```python
from build123d import *

# Parameters (mm, degrees)
SKETCH_1_W          = 100
SKETCH_1_H          = 90
EXTRUDE_1_DEPTH     = 125
SKETCH_4_W          = 100
SKETCH_4_H          = 83
CUT_EXTRUDE_3_DEPTH = 120
FILLET_4_R          = 5
CUT_EXTRUDE_4_DEPTH = 120
SKETCH_6_W          = 23
SKETCH_6_H          = 12.5
CUT_EXTRUDE_5_DEPTH = 2


with BuildPart() as part:
    # 스케치1 → 보스-돌출1 (new body)
    with BuildSketch(Plane(origin=(0, 0, 0), x_dir=(1, 0, 0), z_dir=(0, 1, 0))):
        Rectangle(SKETCH_1_W, SKETCH_1_H)
    extrude(amount=EXTRUDE_1_DEPTH)

    # 스케치4 → 컷-돌출3 (cut)
    with BuildSketch(Plane.XZ):
        with Locations((0, -3.5)):
            Rectangle(SKETCH_4_W, SKETCH_4_H)
    extrude(amount=-CUT_EXTRUDE_3_DEPTH, mode=Mode.SUBTRACT)

    # 필렛4
    fillet_4_edges = [part.edges().sort_by_distance(p)[0] for p in [
        (50, 62.5, 45),
        (-50, 62.5, 45),
        (-50, 122.5, -45),
        (50, 122.5, -45),
    ]]
    fillet(fillet_4_edges, radius=FILLET_4_R)

    # 스케치5 → 컷-돌출4 (cut)
    with BuildSketch(Plane(origin=(0, 0, 38), x_dir=(-1, 0, 0), z_dir=(0, 0, -1))):
        with BuildLine():
            Line((26.25, 63), (28.26707195, 63))
            ThreePointArc((28.26707195, 63), (40, 60), (28.26707195, 57))
            Line((28.26707195, 57), (26.25, 57))
            ThreePointArc((26.25, 57), (23.25, 60), (26.25, 63))
        make_face()
    extrude(amount=-CUT_EXTRUDE_4_DEPTH, mode=Mode.SUBTRACT)

    # 스케치6 → 컷-돌출5 (cut)
    with BuildSketch(Plane(origin=(0, 0, 38), x_dir=(-1, 0, 0), z_dir=(0, 0, -1))):
        with Locations((28.5, 60)):
            Rectangle(SKETCH_6_W, SKETCH_6_H)
    extrude(amount=-CUT_EXTRUDE_5_DEPTH, mode=Mode.SUBTRACT)


solid = part.part
```
For this review, take the finished solid that the model builds, in its own axes (mm). A direction names the side the tool comes from. Round coordinates to 2 decimals unless told otherwise and drop trailing zeros. Order: outer loops, then holes, each group sorted by start corner. A loop starts at its lowest first (then second) coordinate and runs counter-clockwise, first axis right, second up. Notation, with made-up numbers: (37.5, 40.25) -> (73.5, 40.25) arc R38 cw to (73.5, 78.25) -> close; hole circle Ø6 at (43, 15.25). An arc over 180 degrees is marked (long way). Use a Markdown table: item, result.
Item 1: Take a section at B-B (y = 109). State the section outline as (x, z) points, plus the area to 3 significant figures.
Resolved:
| item | result |
|---|---|
| outline | (-50, 38) -> (50, 38) -> (50, 40) arc R5 ccw to (45, 45) -> (-45, 45) arc R5 ccw to (-50, 40) -> close |
| area | 689 mm² |
Item 2: For line 1 along Y through (x, z) = (-33.75, 42.5); line 2 along Z through (x, y) = (27, 17); line 3 along Y through (x, z) = (42, 16.5), list the stretches that pass through material, from the lowest coordinate up. Write a range as [from, to].
Resolved:
| item | result |
|---|---|
| line 1 | y = [0, 53.75], [66.25, 125] |
| line 2 | z = [38, 45] |
| line 3 | y = [120, 125] |
Item 3: Draft analysis for pull direction Y (two halves, no side actions). For faces 5 (the flat face through (-1, 0, 41)), 6 (the flat face through (-22, 60, 40)), 7 (the cylindrical face through (48, 123, -44)), state which applies: +Y half, -Y half, draft (parallel to the pull), parting line (faces both ways), or undercut.
Resolved:
| item | result |
|---|---|
| face 5 | -Y half |
| face 6 | undercut |
| face 7 | draft |
Item 4: Machinability: for faces 1 (the flat face through (-38, 65, 40)), 2 (the cylindrical face through (-49, 123, -43)), 3 (the cylindrical face through (-23.25, 59.93, 42.46)), 4 (the flat face through (-1, 59, 38)), which of the approach directions +Z, -Z, +X, -X, +Y, -Y give a long, thin tool a straight path to every point of the face, cutting with its end or side? Answer none if there is none.
Resolved:
| item | result |
|---|---|
| face 1 | -Z |
| face 2 | -Z, -X, +Y, -Y |
| face 3 | +Z, -Z |
| face 4 | -Z, +X, -X, -Y |
Item 5: Take a section at C-C (z = 15). State the section outline as (x, y) points, plus the area to 3 significant figures.
Resolved:
| item | result |
|---|---|
| outline | (-50, 120) -> (50, 120) -> (50, 125) -> (-50, 125) -> close |
| area | 500 mm² |
Item 6: For pin 1 (3 mm diameter, centred on x = -37.5, y = 57.5, fed in from -Z); pin 2 (4 mm diameter, centred on x = -25.5, y = 58.5, fed in from -Z); pin 3 (1.5 mm diameter, centred on x = 22.5, z = 2, fed in from -Y); pin 4 (2 mm diameter, centred on x = -10, y = 95.5, fed in from -Z), all flat-tipped, find the tip position at first contact; note any pin that passes through.
Resolved:
| item | result |
|---|---|
| pin 1 | passes through |
| pin 2 | stops at z = 40 |
| pin 3 | stops at y = 120 |
| pin 4 | stops at z = 38 |
Item 7: Take a section at A-A (x = 4). State the section outline as (y, z) points.
Resolved:
| item | result |
|---|---|
| outline | (0, 38) -> (120, 38) -> (120, -45) -> (125, -45) -> (125, 45) -> (0, 45) -> close |
